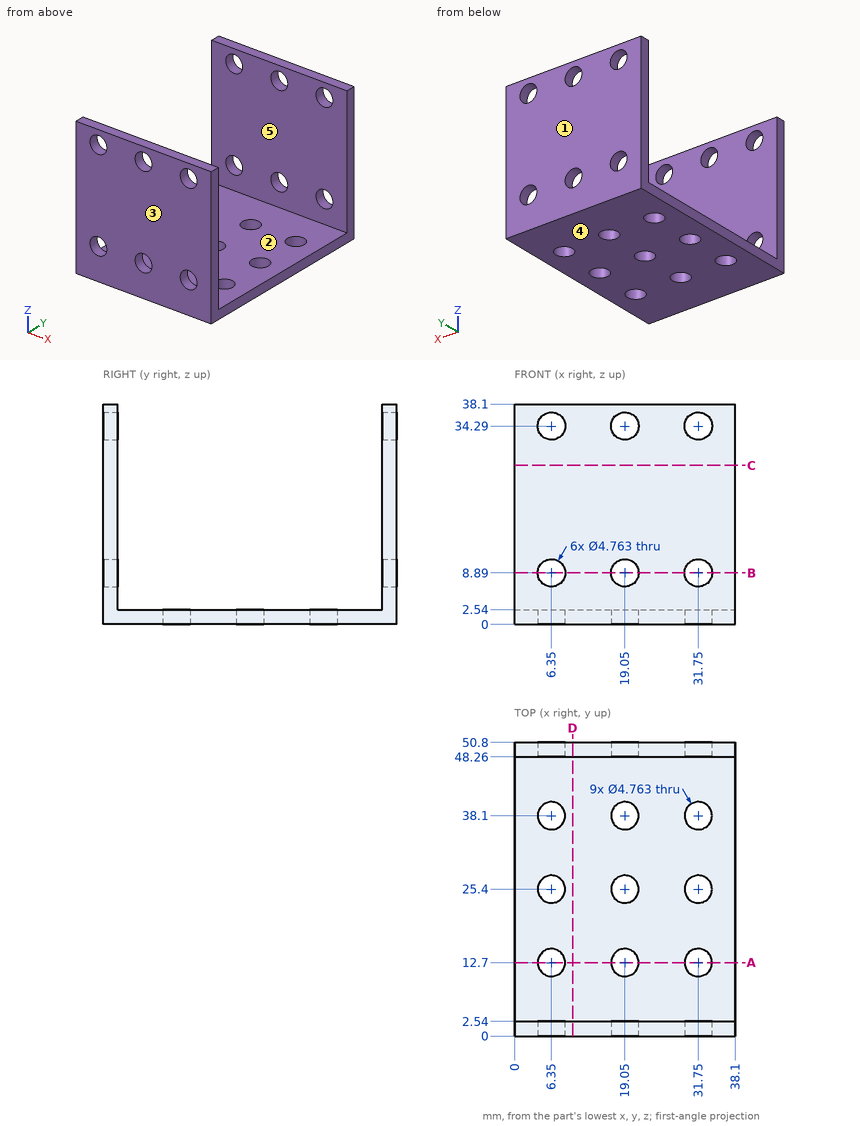
Check sheet for the drawn part. Datum: minimum x, y, z corner. Units: mm. A direction names the side the tool comes from. Round coordinates to 2 decimals unless told otherwise and drop trailing zeros. Order: outer loops, then holes, each group sorted by start corner. A loop starts at its lowest first (then second) coordinate and runs counter-clockwise, first axis right, second up. Notation, with made-up numbers: M 10.25,2 L 52.25,2 A24 ccw 52.25,40 Z; hole C -24.5,9.25 d11. An arc over 180 degrees is marked long. Answer in a Markdown table with one row per item.
(1) Material ranges on line 1 along Z through (x, y) = (31.75, 1); line 2 along Y through (x, z) = (28, 26.5); line 3 along Y through (x, z) = (31, 1), recorded low to high. Write a range as from..to.
Findings:
| item | result |
|---|---|
| line 1 | z = 0..6.51, 11.27..31.91, 36.67..38.1 |
| line 2 | y = 0..2.54, 48.26..50.8 |
| line 3 | y = 0..10.44, 14.96..23.14, 27.66..35.84, 40.36..50.8 |
(2) Section check A-A on y = 12.7. Record the boundary of the cut face in (x, z).
Findings:
| item | result |
|---|---|
| outline | M 0,0 L 3.97,0 L 3.97,2.54 L 0,2.54 Z; M 8.73,0 L 16.67,0 L 16.67,2.54 L 8.73,2.54 Z; M 21.43,0 L 29.37,0 L 29.37,2.54 L 21.43,2.54 Z; M 34.13,0 L 38.1,0 L 38.1,2.54 L 34.13,2.54 Z |
(3) Section check D-D on x = 10. Record the boundary of the cut face in (y, z).
Findings:
| item | result |
|---|---|
| outline | M 0,0 L 50.8,0 L 50.8,38.1 L 48.26,38.1 L 48.26,2.54 L 2.54,2.54 L 2.54,38.1 L 0,38.1 Z |
(4) Section check B-B on z = 8.89. Give the number of separate pieces and of enclosed holes in the cut face, plus the area to 3 significant figures.
Findings:
| item | result |
|---|---|
| separate pieces | 8 |
| enclosed holes | 0 |
| area | 121 mm^2 |
(5) Gauge pin test, flat ends, axial feed: pin 1 (6 mm diameter, centred on y = 23, z = 7, fed in from +X); pin 2 (6 mm diameter, centred on x = 6.35, z = 34.29, fed in from +Y); pin 3 (6 mm diameter, centred on x = 31.75, y = 38.1, fed in from +Z). Record the tip position at first contact, or that the pin passes through.
Findings:
| item | result |
|---|---|
| pin 1 | passes through |
| pin 2 | stops at y = 50.8 |
| pin 3 | stops at z = 2.54 |
(6) Draft check along Y on the marked faces 1, 2 and 3. Enter one of: +Y half, -Y half, draft (parallel to the pull), parting line (faces both ways), or undercut.
Findings:
| item | result |
|---|---|
| face 1 | +Y half |
| face 2 | undercut |
| face 3 | -Y half |
(7) Set-up check for the marked faces 4 and 5: record each of +Z, -Z, +X, -X, +Y, -Y from which the full face is reachable in a straight line by a thin tool's end or side.
Findings:
| item | result |
|---|---|
| face 4 | -Z, +X, -X, +Y, -Y |
| face 5 | +Z, +X, -X |
(8) Section check C-C on z = 27.5. Record the boundary of the cut face in (x, y).
Findings:
| item | result |
|---|---|
| outline | M 0,0 L 38.1,0 L 38.1,2.54 L 0,2.54 Z; M 0,48.26 L 38.1,48.26 L 38.1,50.8 L 0,50.8 Z |
